Could you check a few things on this model? Use its own coordinates, in mm. A direction names the side the tool comes from. Give positions to 0.01 mm unless a question says otherwise; leave off trailing zeros. Write each loop counter-clockwise with the first axis right and the second up, starting at its lowest first coordinate (ties: lowest second). Pieces come first, ordered by that corner, then holes. Notation, with made-up numbers: (77.25, 32.25) - (115.25, 32.25) arc R25 cw to (115.25, 66.25) - close; hole circle Ø1 at (85, -32). An arc over 180 degrees is marked (long way). Answer as CSV lines item,"result". Start each with the question number.
Q1. Imagine slicing it at D-D on x = -17.5. List the corners of the cut face in (y, z) for me.
Q2. Imagine slicing it at B-B on z = 0. List the corners of the cut face in (x, y) for me.
Q3. On a 3-axis mill with a long thin cutter (end or side, diameter ignored), from which of +Z, -Z, +X, -X, +Y, -Y can I reach the whole of each face in a straight line? I mean faces 5 (the face through (-22, 25, 12.5)), 6 (the face through (2.5, -47, 0)), 7 (the face through (-15, -56, 6)), 8 (the face through (15, -56, 6)). Say none if no direction works.
Q4. We'd pull the mould along Y, two halves only. Please class faces 1 (the face through (1, 58.5, 0)), 2 (the face through (-22, 25, -12.5)), 3 (the face through (9, -66.122, 0)), 4 (the face through (-8.84, -61.2, -2.11)): pulls with the +Y half, pulls with the -Y half, needs draft (parallel to the pull), parting line crosses it, or undercut.
Q5. Imagine slicing it at A-A on x = 10. List the corners of the cut face in (y, z) for me, and give its area (3 significant figures).
Q6. Imagine slicing it at C-C on y = -8.5. List the corners of the cut face in (x, z) for me.
Q7. If I drill on line 1 along Y through (x, z) = (-12, -5); line 2 along Y through (x, z) = (-3.5, -9); line 3 along Y through (x, z) = (0, -0.5), over which ranges is the centre line in solid material (lowest first)?
Q8. Will these pins go through, and if not, where does the flat tip stop? pin 1 Ø2 at (y, z) = (-21.5, 8.5) entering from -X; pin 2 Ø12.5 at (y, z) = (-56.12, 0) entering from -X; pin 3 Ø8 at (y, z) = (-22, 8.5) entering from -X.
```python
from build123d import *

# Parameters (mm, degrees)
F1_DEPTH = 12.5
F3_D     = 11


with BuildPart() as f1:
    # F0 (on Top) → F1 (new body, symmetric)
    with BuildSketch(Plane.XY):
        with BuildLine():
            ThreePointArc((28.5, 0), (21.017849557, -19.2483765549), (2.5, -28.3901391332))
            Line((2.5, -28.3901391332), (2.5, -66.1221205063))
            Line((2.5, -66.1221205063), (15, -66.1221205063))
            Line((15, -66.1221205063), (15, -46.1221205063))
            ThreePointArc((15, -46.1221205063), (39.2412410609, -28.5021928981), (48.5, 0))
            Line((48.5, 0), (28.5, 0))
        make_face()
        with BuildLine():
            ThreePointArc((-28.5, 0), (0, 28.5), (28.5, 0))
            Line((28.5, 0), (48.5, 0))
            ThreePointArc((48.5, 0), (0, 48.5), (-48.5, 0))
            Line((-48.5, 0), (-28.5, 0))
        make_face()
        with BuildLine():
            ThreePointArc((-2.5, -28.3901391332), (-21.017849557, -19.2483765549), (-28.5, 0))
            Line((-28.5, 0), (-48.5, 0))
            ThreePointArc((-48.5, 0), (-39.2412410609, -28.5021928981), (-15, -46.1221205063))
            Line((-15, -46.1221205063), (-15, -66.1221205063))
            Line((-15, -66.1221205063), (-2.5, -66.1221205063))
            Line((-2.5, -66.1221205063), (-2.5, -28.3901391332))
        make_face()
        with BuildLine():
            ThreePointArc((-48.5, 0), (0, 48.5), (48.5, 0))
            Line((48.5, 0), (48.5, 58.5))
            Line((48.5, 58.5), (-48.5, 58.5))
            Line((-48.5, 58.5), (-48.5, 0))
        make_face()
    extrude(amount=F1_DEPTH, both=True)

    # F3 (through all)
    with Locations(Plane.YZ.offset(15)):
        with Locations((-56.1221205063, 0)):
            Hole(F3_D / 2)


solid = f1.part
```
Conclusion:
1,outline,"(-45.23, -12.5) - (-22.49, -12.5) - (-22.49, 12.5) - (-45.23, 12.5) - close; (22.49, -12.5) - (58.5, -12.5) - (58.5, 12.5) - (22.49, 12.5) - close"
2,outline,"(-48.5, 0) arc R48.5 ccw to (-15, -46.12) - (-15, -50.62) - (-2.5, -50.62) - (-2.5, -28.39) arc R28.5 cw (long way) to (2.5, -28.39) - (2.5, -50.62) - (15, -50.62) - (15, -46.12) arc R48.5 ccw to (48.5, 0) - (48.5, 58.5) - (-48.5, 58.5) - close; (-15, -66.12) - (-2.5, -66.12) - (-2.5, -61.62) - (-15, -61.62) - close; (2.5, -66.12) - (15, -66.12) - (15, -61.62) - (2.5, -61.62) - close"
3,face 5,"+Z, +X, -X, +Y, -Y"
3,face 6,"+Z, -Z, -Y"
3,face 7,"+Z, -Z, -X, -Y"
3,face 8,"+Z, -Z, +X, -Y"
4,face 1,"pulls with the +Y half"
4,face 2,"needs draft"
4,face 3,"pulls with the -Y half"
4,face 4,"undercut"
5,outline,"(-66.12, -12.5) - (-26.69, -12.5) - (-26.69, 12.5) - (-66.12, 12.5) - close; (26.69, -12.5) - (58.5, -12.5) - (58.5, 12.5) - (26.69, 12.5) - close; hole circle Ø11 at (-56.12, 0)"
5,area,"1,690 mm^2"
6,outline,"(-47.75, -12.5) - (-27.2, -12.5) - (-27.2, 12.5) - (-47.75, 12.5) - close; (27.2, -12.5) - (47.75, -12.5) - (47.75, 12.5) - (27.2, 12.5) - close"
7,line 1,"-66.12 to -58.41, -53.83 to -25.85, 25.85 to 58.5"
7,line 2,"-66.12 to -28.28, 28.28 to 58.5"
7,line 3,"28.5 to 58.5"
8,pin 1,"x = -43.95"
8,pin 2,"x = -15"
8,pin 3,"x = -45.04"
